```python
from build123d import *

# Parameters (mm, degrees)
F0_W     = 889
F0_H     = 1498.6
F1_DEPTH = 609.6
F2_W     = 685.8
F2_H     = 1295.4
F3_DEPTH = 508
F4_R     = 76.2
F5_R     = 76.2
F6_R     = 76.2
F7_R     = 76.2
F9_D     = 60.96
F11_D    = 60.96


with BuildPart() as f1:
    # F0 (on Top) → F1 (new body)
    with BuildSketch(Plane.XY):
        with Locations((-594.257204, -16.040897)):
            Rectangle(F0_W, F0_H)
    extrude(amount=F1_DEPTH)

    # F2 (on face) → F3 (cut)
    with BuildSketch(Plane.XY.offset(609.6)):
        with Locations((-594.257204, -16.040897)):
            Rectangle(F2_W, F2_H)
    extrude(amount=-F3_DEPTH, mode=Mode.SUBTRACT)

    # F4
    f4_edges = [f1.edges().sort_by_distance(p)[0] for p in [
        (-937.157204, 631.659103, 355.6),
    ]]
    fillet(f4_edges, radius=F4_R)

    # F5
    f5_edges = [f1.edges().sort_by_distance(p)[0] for p in [
        (-251.357204, 631.659103, 355.6),
    ]]
    fillet(f5_edges, radius=F5_R)

    # F6
    f6_edges = [f1.edges().sort_by_distance(p)[0] for p in [
        (-251.357204, -663.740897, 355.6),
    ]]
    fillet(f6_edges, radius=F6_R)

    # F7
    f7_edges = [f1.edges().sort_by_distance(p)[0] for p in [
        (-937.157204, -663.740897, 355.6),
    ]]
    fillet(f7_edges, radius=F7_R)

    # F9 (through all)
    with Locations(Plane.XZ.offset(-631.659103)):
        with Locations((-594.257204, 508)):
            Hole(F9_D / 2)

    # F11 (through all)
    with Locations(Plane(origin=(0, -663.740897, 0), x_dir=(-1, 0, 0), z_dir=(0, 1, 0))):
        with Locations((594.257204, 508)):
            Hole(F11_D / 2)


solid = f1.part
```
The listing builds one solid part. Answer for the finished solid, in the listing's coordinates (mm). A direction names the side the tool comes from. Give positions to 0.01 mm unless a question says otherwise; leave off trailing zeros. Write each loop counter-clockwise with the first axis right and the second up, starting at its lowest first coordinate (ties: lowest second). Pieces come first, ordered by that corner, then holes. Notation, with made-up numbers: (34, -30.75) -> (61, -30.75) arc R20 ccw to (61, -7.75) -> close; hole circle Ø9 at (-27, 15). An arc over 180 degrees is marked (long way). Write item = value, one per line. Start each with the question number.
1) The part is cut by section B-B, the plane x = -664.5. Determine the outline of the cut face in (y, z).
2) This flat-tipped pin is pushed along its axis until it touches: pin 1 (2 mm diameter, centred on x = -533, y = -365.5, fed in from +Z). Where does it stop, or does it pass through?
3) The part is cut by section C-C, the plane z = 336.5. Determine the outline of the cut face in (x, y), and give its area (3 significant figures).
4) Determine the mould class of faces 1 (the face through (-914.243, -642.012, 352.044)), 2 (the face through (-1038.757, -27, 301)), 3 (the face through (-996, -6, 609.6)) for opening direction X: +X half, -X half, draft (parallel to the pull), parting line (faces both ways), or undercut.
5) Straight lines are drawn through the part: line 1 along Y through (x, z) = (-553.5, 431); line 2 along X through (y, z) = (-699, 508); line 3 along Y through (x, z) = (-864, 245.5). For each, find the intervals that lie inside material, in ascending order.
6) The part is cut by section D-D, the plane y = -540. Determine the outline of the cut face in (x, z).
7) The part is cut by section A-A, the plane z = 508. Determine the outline of the cut face in (x, y), and give its area (3 significant figures).
8) Which of the six approach directions +Z, -Z, +X, -X, +Y, -Y give full straight-line access (tool end or side, diameter ignored) to faces 4 (the face through (-600, -765.341, 301)), 5 (the face through (-273.09, -640.83, 352.04))?
Solutions:
q1.outline = (-765.34, 0) -> (733.26, 0) -> (733.26, 609.6) -> (631.66, 609.6) -> (631.66, 101.6) -> (-663.74, 101.6) -> (-663.74, 609.6) -> (-765.34, 609.6) -> close
q2.pin_1 = 101.6
q3.outline = (-1038.76, -765.34) -> (-149.76, -765.34) -> (-149.76, 733.26) -> (-1038.76, 733.26) -> close; hole (-937.16, -587.54) arc R76.2 ccw to (-860.96, -663.74) -> (-327.56, -663.74) arc R76.2 ccw to (-251.36, -587.54) -> (-251.36, 555.46) arc R76.2 ccw to (-327.56, 631.66) -> (-860.96, 631.66) arc R76.2 ccw to (-937.16, 555.46) -> close
q3.area = 449,000 mm²
q4.face_1 = undercut
q4.face_2 = -X half
q4.face_3 = draft
q5.line_1 = -765.34 to -663.74, 631.66 to 733.26
q5.line_2 = -1038.76 to -624.74, -563.78 to -149.76
q5.line_3 = -765.34 to -663.68, 631.6 to 733.26
q6.outline = (-1038.76, 0) -> (-149.76, 0) -> (-149.76, 609.6) -> (-251.36, 609.6) -> (-251.36, 101.6) -> (-937.16, 101.6) -> (-937.16, 609.6) -> (-1038.76, 609.6) -> close
q7.outline = (-1038.76, -765.34) -> (-624.74, -765.34) -> (-624.74, -663.74) -> (-860.96, -663.74) arc R76.2 cw to (-937.16, -587.54) -> (-937.16, 555.46) arc R76.2 cw to (-860.96, 631.66) -> (-624.74, 631.66) -> (-624.74, 733.26) -> (-1038.76, 733.26) -> close; (-563.78, -765.34) -> (-149.76, -765.34) -> (-149.76, 733.26) -> (-563.78, 733.26) -> (-563.78, 631.66) -> (-327.56, 631.66) arc R76.2 cw to (-251.36, 555.46) -> (-251.36, -587.54) arc R76.2 cw to (-327.56, -663.74) -> (-563.78, -663.74) -> close
q7.area = 436,000 mm²
q8.face_4 = +Z, -Z, +X, -X, -Y
q8.face_5 = +Z
